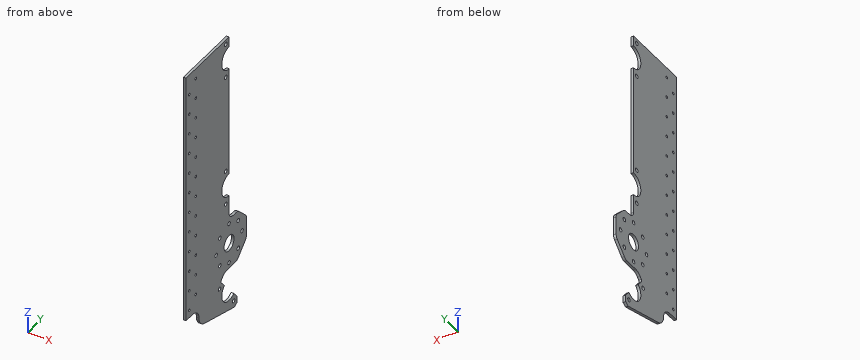
```python
from build123d import *

# Parameters (mm, degrees)
SKETCH1_R                  = 9.779
SKETCH1_R_2                = 2.413
BOSS_EXTRUDE1_DEPTH        = 3.175
F_10_CLEARANCE_HOLE1_D     = 4.9784
F_10_CLEARANCE_HOLE2_D     = 4.9784
F_10_CLEARANCE_HOLE2_DEPTH = 3.175
F_10_CLEARANCE_HOLE2_TIP   = 1.495662253
CHAMFER1_SIZE              = 5.08
CHAMFER1_SIZE2             = 4.1342197
FILLET1_R                  = 7.62
SKETCH7_R                  = 1.5875
CUT_EXTRUDE1_DEPTH         = 346.209763321


with BuildPart() as part:
    # Sketch1 → Boss-Extrude1 (new body)
    with BuildSketch(Plane(origin=(0, 0, 0), x_dir=(0, 0, -1), z_dir=(1, 0, 0))):
        with BuildLine():
            Line((-12.7, -12.7), (-328.6379, -12.7))
            Line((-328.6379, -12.7), (-328.6379, 71.4629))
            Line((-328.6379, 71.4629), (-315.9379, 71.4629))
            ThreePointArc((-315.9379, 71.4629), (-301.625, 57.15), (-287.3121, 71.4629))
            Line((-287.3121, 71.4629), (-150.8125, 71.4629))
            ThreePointArc((-150.8125, 71.4629), (-136.4996, 57.15), (-122.1867, 71.4629))
            Line((-122.1867, 71.4629), (-91.313, 71.4629))
            Line((-91.313, 71.4629), (-91.313, 88.788677931))
            Line((-91.313, 88.788677931), (-74.475777931, 105.6259))
            Line((-74.475777931, 105.6259), (-46.174222069, 105.6259))
            Line((-46.174222069, 105.6259), (-27.855333333, 87.307011265))
            Line((-27.855333333, 87.307011265), (-27.855333333, 67.615437998))
            ThreePointArc((-27.855333333, 67.615437998), (-26.836905275, 62.632379001), (-23.944959008, 58.448514823))
            Line((-23.944959008, 58.448514823), (-21.653228214, 56.251108404))
            ThreePointArc((-21.653228214, 56.251108404), (-19.979435171, 55.545886769), (-18.262622551, 56.138740153))
            Line((-18.262622551, 56.138740153), (-10.96431751, 62.262745221))
            ThreePointArc((-10.96431751, 62.262745221), (9.200154779, 60.49858249), (10.96431751, 80.663054779))
            Line((10.96431751, 80.663054779), (18.262622551, 86.787059847))
            Line((18.262622551, 86.787059847), (30.962622551, 86.787059847))
            Line((30.962622551, 86.787059847), (13.473085073, 22.977185543))
            ThreePointArc((13.473085073, 22.977185543), (8.472670241, 15.562580904), (0, 12.7))
            ThreePointArc((0, 12.7), (-8.980256121, 8.980256121), (-12.7, 0))
            Line((-12.7, 0), (-12.7, -12.7))
        make_face()
        with Locations((-60.325, 71.4629)):
            Circle(SKETCH1_R, mode=Mode.SUBTRACT)
        with Locations((-60.325, 96.8629)):
            Circle(SKETCH1_R_2, mode=Mode.SUBTRACT)
        with Locations((-42.364487758, 89.423412242)):
            Circle(SKETCH1_R_2, mode=Mode.SUBTRACT)
        with Locations((-34.925, 71.4629)):
            Circle(SKETCH1_R_2, mode=Mode.SUBTRACT)
        with Locations((-42.364487758, 53.502387758)):
            Circle(SKETCH1_R_2, mode=Mode.SUBTRACT)
        with Locations((-60.325, 46.0629)):
            Circle(SKETCH1_R_2, mode=Mode.SUBTRACT)
        with Locations((-78.285512242, 53.502387758)):
            Circle(SKETCH1_R_2, mode=Mode.SUBTRACT)
        with Locations((-85.725, 71.4629)):
            Circle(SKETCH1_R_2, mode=Mode.SUBTRACT)
        with Locations((-78.285512242, 89.423412242)):
            Circle(SKETCH1_R_2, mode=Mode.SUBTRACT)
    extrude(amount=BOSS_EXTRUDE1_DEPTH)

    # #10 Clearance Hole1 (through all)
    with Locations(Plane(origin=(3.175, 0, 0), x_dir=(0, 0, -1), z_dir=(1, 0, 0))):
        with Locations((-323.05625, 65.1129), (-280.19375, 65.1129), (-157.93085, 65.1129), (-115.06835, 65.1129), (-12.33558865, 52.822775826), (20.498991293, 80.374259746)):
            Hole(F_10_CLEARANCE_HOLE1_D / 2)

    # #10 Clearance Hole2
    with Locations(Plane(origin=(3.175, 0, 0), x_dir=(0, 0, -1), z_dir=(1, 0, 0))):
        with Locations((-60.325, 96.8629), (-42.364487758, 89.423412242), (-34.925, 71.4629), (-42.364487758, 53.502387758), (-60.325, 46.0629), (-78.285512242, 53.502387758), (-85.725, 71.4629), (-78.285512242, 89.423412242)):
            Hole(F_10_CLEARANCE_HOLE2_D / 2, depth=F_10_CLEARANCE_HOLE2_DEPTH)
            with Locations((0, 0, -(F_10_CLEARANCE_HOLE2_DEPTH + F_10_CLEARANCE_HOLE2_TIP / 2))):  # 118° drill point
                Cone(0, F_10_CLEARANCE_HOLE2_D / 2, F_10_CLEARANCE_HOLE2_TIP, mode=Mode.SUBTRACT)

    # Chamfer1
    chamfer1_edges = [part.edges().sort_by_distance(p)[0] for p in [
        (1.5875, 86.787059847, -30.962622551),
    ]]
    chamfer1_side = [part.faces().sort_by_distance(p)[0] for p in [
        (1.5875, 54.882122695, -22.217853812),
    ]]
    chamfer(chamfer1_edges, length=CHAMFER1_SIZE, length2=CHAMFER1_SIZE2, reference=chamfer1_side[0])

    # Fillet1
    fillet1_edges = [part.edges().sort_by_distance(p)[0] for p in [
        (1.5875, 71.4629, 91.313),
        (1.5875, 88.788677931, 91.313),
        (1.5875, 105.6259, 74.475777931),
        (1.5875, 105.6259, 46.174222069),
        (1.5875, 87.307011265, 27.855333333),
    ]]
    fillet(fillet1_edges, radius=FILLET1_R)

    # Sketch7 → Cut-Extrude1 (cut, through all)
    with BuildSketch(Plane.ZY):
        with Locations((315.9379, 6.35)):
            Circle(SKETCH7_R)
        with Locations((303.2379, -6.35)):
            Circle(SKETCH7_R)
        with Locations((290.393581818, 6.35)):
            Circle(SKETCH7_R)
        with Locations((277.693581818, -6.35)):
            Circle(SKETCH7_R)
        with Locations((264.849263636, 6.35)):
            Circle(SKETCH7_R)
        with Locations((252.149263636, -6.35)):
            Circle(SKETCH7_R)
        with Locations((239.304945455, 6.35)):
            Circle(SKETCH7_R)
        with Locations((226.604945455, -6.35)):
            Circle(SKETCH7_R)
        with Locations((213.760627273, 6.35)):
            Circle(SKETCH7_R)
        with Locations((201.060627273, -6.35)):
            Circle(SKETCH7_R)
        with Locations((188.216309091, 6.35)):
            Circle(SKETCH7_R)
        with Locations((175.516309091, -6.35)):
            Circle(SKETCH7_R)
        with Locations((162.671990909, 6.35)):
            Circle(SKETCH7_R)
        with Locations((149.971990909, -6.35)):
            Circle(SKETCH7_R)
        with Locations((137.127672727, 6.35)):
            Circle(SKETCH7_R)
        with Locations((124.427672727, -6.35)):
            Circle(SKETCH7_R)
        with Locations((111.583354545, 6.35)):
            Circle(SKETCH7_R)
        with Locations((98.883354545, -6.35)):
            Circle(SKETCH7_R)
        with Locations((86.039036364, 6.35)):
            Circle(SKETCH7_R)
        with Locations((73.339036364, -6.35)):
            Circle(SKETCH7_R)
        with Locations((60.494718182, 6.35)):
            Circle(SKETCH7_R)
        with Locations((47.794718182, -6.35)):
            Circle(SKETCH7_R)
        with Locations((34.9504, 6.35)):
            Circle(SKETCH7_R)
        with Locations((22.2504, -6.35)):
            Circle(SKETCH7_R)
    extrude(amount=-CUT_EXTRUDE1_DEPTH, mode=Mode.SUBTRACT)


solid = part.part
```
Geometry check sheet. Reference: the model listing, model coordinates, mm. Coordinates: 2 decimals unless noted, no trailing zeros. Order: outer loops, then holes, each group sorted by start corner. A loop starts at its lowest first (then second) coordinate and runs counter-clockwise, first axis right, second up.
Item 1: Section check B-B (x = 1.35). Count the separate pieces of the cut face and the enclosed holes in it, plus the area to 3 significant figures.
Item 2: Section check A-A (z = 54). Enter the section's corners in (x, y) (3 decimals), plus the area to 3 significant figures.
Item 3: Scan lines: line 1 along Y through (x, z) = (1.55, 42.5); line 2 along Z through (x, y) = (0.25, -3.5); line 3 along Y through (x, z) = (0.65, 125). Record each from-to range of solid material in increasing order.
Item 4: Depth check by flat-ended pin: pin 1 (1.6 mm diameter, centred on x = 2.5, z = -24.5, fed in from +Y); pin 2 (1 mm diameter, centred on x = 1.5, z = 114.5, fed in from +Y). Enter the tip coordinate at first touch or a pass-through.
Check sheet entries:
1. separate pieces: 1
1. enclosed holes: 39
1. area: 28,600 mm2
2. outline: (0, -12.7) - (3.175, -12.7) - (3.175, 64.005) - (0, 64.005) - close; (0, 78.921) - (3.175, 78.921) - (3.175, 105.626) - (0, 105.626) - close
2. area: 328 mm2
3. line 1: y = -12.7 to 51.02, 55.99 to 86.94, 91.91 to 101.95
3. line 2: z = 12.7 to 328.64
3. line 3: y = -12.7 to -7.83, -4.87 to 62.94
4. pin 1: stops at y = 86.79
4. pin 2: stops at y = 71.46
